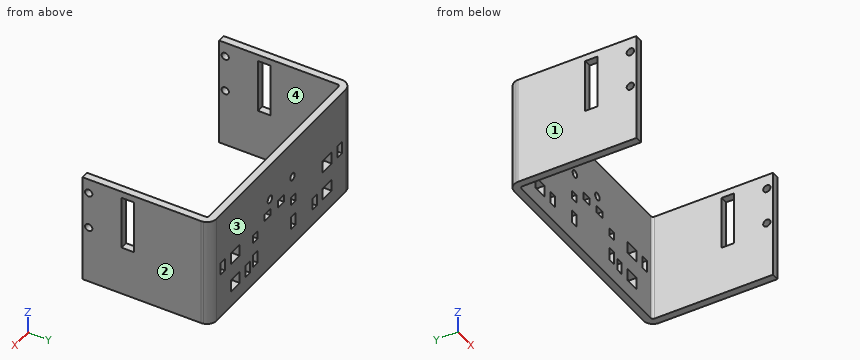
from build123d import *

# Parameters (mm, degrees)
SKETCH1_R                  = 1.5
SKETCH1_W                  = 2.9
SKETCH1_H                  = 5
SKETCH1_W_2                = 6
SKETCH1_W_3                = 5
SKETCH1_H_2                = 22
BASE_FLANGE1_DEPTH         = 3
SKETCH34_W                 = 3
SKETCH34_H                 = 5.190452684
SKETCH34_H_2               = 3.298760194
CUT_EXTRUDE2_DEPTH         = 10
SKETCH35_W                 = 4
SKETCH35_H                 = 3
CUT_EXTRUDE3_DEPTH         = 10
SKETCHED_START             = -31.946571622
SKETCHED_BEND1_DEPTH       = 45
SKETCHED_BEND1_2_OUTLINE_W = 3
SKETCHED_BEND1_2_OUTLINE_H = 16
SKETCHED_BEND1_2_DEPTH     = 45
SKETCHED_BEND1_3_OUTLINE_W = 3
SKETCHED_BEND1_3_OUTLINE_H = 5
SKETCHED_BEND1_3_DEPTH     = 20.3
SKETCHED_START_2           = 10.353428378
SKETCHED_BEND1_4_OUTLINE_W = 3
SKETCHED_BEND1_4_OUTLINE_H = 5
SKETCHED_BEND1_4_DEPTH     = 2.7
SKETCHED_START_3           = -48
SKETCHED_BEND1_5_OUTLINE_R = 1.5
SKETCHED_BEND1_5_DEPTH     = 96


with BuildPart() as part:
    # Base-Flange1: sheet metal written as solids
    # Sketch1 → Base-Flange1 (new body)
    with BuildSketch(Plane(origin=(0, 0, 0), x_dir=(1, 0, 0), z_dir=(0, 1, 0))):
        Polygon((-95, 31.946571622), (-95, -13.053428378), (95, -13.053428378), (95, 31.946571622), (45, 31.946571622), (-45, 31.946571622), align=None)
        with Locations(Location((92.5, -7.053428378, 0), (0, 0, 270))):
            Circle(SKETCH1_R, mode=Mode.SUBTRACT)
        with Locations(Location((92.5, 8.146571622, 0), (0, 0, 270))):
            Circle(SKETCH1_R, mode=Mode.SUBTRACT)
        with Locations(Location((-92.5, -7.053428378, 0), (0, 0, 90))):
            Circle(SKETCH1_R, mode=Mode.SUBTRACT)
        with Locations(Location((-92.5, 8.146571622, 0), (0, 0, 90))):
            Circle(SKETCH1_R, mode=Mode.SUBTRACT)
        with Locations(Location((7.6, 1.946571622, 0), (0, 0, 270))):
            Circle(SKETCH1_R, mode=Mode.SUBTRACT)
        with Locations(Location((-7.6, 1.946571622, 0), (0, 0, 270))):
            Circle(SKETCH1_R, mode=Mode.SUBTRACT)
        with Locations((-39.45, 10.905641405)):
            Rectangle(SKETCH1_W, SKETCH1_H, mode=Mode.SUBTRACT)
        with Locations((-22.55, 22.947848405)):
            Rectangle(SKETCH1_W, SKETCH1_H, mode=Mode.SUBTRACT)
        with Locations((-31, 22.946571622)):
            Rectangle(SKETCH1_W_2, SKETCH1_H, mode=Mode.SUBTRACT)
        with Locations((-31, 10.946571622)):
            Rectangle(SKETCH1_W_2, SKETCH1_H, mode=Mode.SUBTRACT)
        with Locations((31, 10.946571622)):
            Rectangle(SKETCH1_W_2, SKETCH1_H, mode=Mode.SUBTRACT)
        with Locations((31, 22.946571622)):
            Rectangle(SKETCH1_W_2, SKETCH1_H, mode=Mode.SUBTRACT)
        with Locations((22.55, 22.947848405)):
            Rectangle(SKETCH1_W, SKETCH1_H, mode=Mode.SUBTRACT)
        with Locations((39.45, 10.905641405)):
            Rectangle(SKETCH1_W, SKETCH1_H, mode=Mode.SUBTRACT)
        with Locations((76.5, 0.646571622)):
            Rectangle(SKETCH1_W_3, SKETCH1_H_2, mode=Mode.SUBTRACT)
        with Locations((-76.5, 0.646571622)):
            Rectangle(SKETCH1_W_3, SKETCH1_H_2, mode=Mode.SUBTRACT)
    extrude(amount=-BASE_FLANGE1_DEPTH)

    # Sketch34 → Cut-Extrude2 (cut)
    with BuildSketch(Plane.XZ.offset(3)):
        with Locations((17.4, -21.824895141)):
            Rectangle(SKETCH34_W, SKETCH34_H)
        with Locations((-8.1, -21.824895141)):
            Rectangle(SKETCH34_W, SKETCH34_H)
        with Locations((-8.1, -12.169238167)):
            Rectangle(SKETCH34_W, SKETCH34_H_2)
        with Locations((17.4, -12.169238167)):
            Rectangle(SKETCH34_W, SKETCH34_H_2)
    extrude(amount=-CUT_EXTRUDE2_DEPTH, mode=Mode.SUBTRACT)

    # Sketch35 → Cut-Extrude3 (cut)
    with BuildSketch(Plane(origin=(0, 0, 0), x_dir=(1, 0, 0), z_dir=(0, 1, 0))):
        with Locations((0.15, 7.74985807)):
            Rectangle(SKETCH35_W, SKETCH35_H)
        with Locations((9.15, 7.806187778)):
            Rectangle(SKETCH35_W, SKETCH35_H)
    extrude(amount=-CUT_EXTRUDE3_DEPTH, mode=Mode.SUBTRACT)

    # Sketched Bend1: read off the stored shape, not the designer's step
    # Sketched Bend1 outline → Sketched Bend1 (cut)
    with BuildSketch(Plane.XY.offset(SKETCHED_START)):
        with BuildLine():
            ThreePointArc((43.5, 0), (45.949489743, -0.83772234), (47.372983346, -3))
            Line((47.372983346, -3), (95, -3))
            Line((95, -3), (95, 0))
            Line((95, 0), (43.5, 0))
        make_face()
        with BuildLine():
            ThreePointArc((-47.372983346, -3), (-45.949489743, -0.83772234), (-43.5, 0))
            Line((-43.5, 0), (-95, 0))
            Line((-95, 0), (-95, -3))
            Line((-95, -3), (-47.372983346, -3))
        make_face()
    extrude(amount=SKETCHED_BEND1_DEPTH, mode=Mode.SUBTRACT)

    # Sketched Bend1 2 outline → Sketched Bend1 2 (add)
    with BuildSketch(Plane.XY.offset(SKETCHED_START)):
        with BuildLine():
            ThreePointArc((43.5, -3), (44.207106781, -3.292893219), (44.5, -4))
            Line((44.5, -4), (44.5, -31.5))
            Line((44.5, -31.5), (47.5, -31.5))
            Line((47.5, -31.5), (47.5, -4))
            ThreePointArc((47.5, -4), (47.468118785, -3.49598283), (47.372983346, -3))
            Line((47.372983346, -3), (43.5, -3))
        make_face()
        with BuildLine():
            ThreePointArc((-44.5, -4), (-44.207106781, -3.292893219), (-43.5, -3))
            Line((-43.5, -3), (-47.372983346, -3))
            ThreePointArc((-47.372983346, -3), (-47.468118785, -3.49598283), (-47.5, -4))
            Line((-47.5, -4), (-47.5, -31.5))
            Line((-47.5, -31.5), (-44.5, -31.5))
            Line((-44.5, -31.5), (-44.5, -4))
        make_face()
        with Locations((46, -44.5)):
            Rectangle(SKETCHED_BEND1_2_OUTLINE_W, SKETCHED_BEND1_2_OUTLINE_H)
        with Locations((-46, -44.5)):
            Rectangle(SKETCHED_BEND1_2_OUTLINE_W, SKETCHED_BEND1_2_OUTLINE_H)
    extrude(amount=SKETCHED_BEND1_2_DEPTH)

    # Sketched Bend1 3 outline → Sketched Bend1 3 (add)
    with BuildSketch(Plane.XY.offset(SKETCHED_START)):
        with Locations((46, -34)):
            Rectangle(SKETCHED_BEND1_3_OUTLINE_W, SKETCHED_BEND1_3_OUTLINE_H)
        with Locations((-46, -34)):
            Rectangle(SKETCHED_BEND1_3_OUTLINE_W, SKETCHED_BEND1_3_OUTLINE_H)
    extrude(amount=SKETCHED_BEND1_3_DEPTH)

    # Sketched Bend1 4 outline → Sketched Bend1 4 (add)
    with BuildSketch(Plane.XY.offset(SKETCHED_START_2)):
        with Locations((46, -34)):
            Rectangle(SKETCHED_BEND1_4_OUTLINE_W, SKETCHED_BEND1_4_OUTLINE_H)
        with Locations((-46, -34)):
            Rectangle(SKETCHED_BEND1_4_OUTLINE_W, SKETCHED_BEND1_4_OUTLINE_H)
    extrude(amount=SKETCHED_BEND1_4_DEPTH)

    # Sketched Bend1 5 outline → Sketched Bend1 5 (cut)
    with BuildSketch(Plane.YZ.offset(SKETCHED_START_3)):
        with Locations((-50, -8.146571622)):
            Circle(SKETCHED_BEND1_5_OUTLINE_R)
        with Locations((-50, 7.053428378)):
            Circle(SKETCHED_BEND1_5_OUTLINE_R)
    extrude(amount=SKETCHED_BEND1_5_DEPTH, mode=Mode.SUBTRACT)


solid = part.part
CAD build for the part. Positions are in the model's coordinates, mm. Face numbers are marked on the shaded views. Coordinates: 2 decimals unless noted, no trailing zeros. Loops run counter-clockwise (first coordinate to the right, second up) from the corner with the lowest first, then second, coordinate; pieces in that order, holes last. Notation, with made-up numbers: (-34.5, 84) -> (-19.5, 84) arc R14 cw to (-19.5, 107) -> close; hole circle Ø10 at (74.25, 89.5). An arc over 180 degrees is marked (long way). One line per item, written item: value.
1. Slice it at B-B on y = -50. Write the cut outline in (x, z), and give its area (3 significant figures).
Answers:
outline: (-47.5, -31.95) -> (-44.5, -31.95) -> (-44.5, -9.65) -> (-47.5, -9.65) -> close; (-47.5, -6.65) -> (-44.5, -6.65) -> (-44.5, 5.55) -> (-47.5, 5.55) -> close; (-47.5, 8.55) -> (-44.5, 8.55) -> (-44.5, 13.05) -> (-47.5, 13.05) -> close; (44.5, -31.95) -> (47.5, -31.95) -> (47.5, -9.65) -> (44.5, -9.65) -> close; (44.5, -6.65) -> (47.5, -6.65) -> (47.5, 5.55) -> (44.5, 5.55) -> close; (44.5, 8.55) -> (47.5, 8.55) -> (47.5, 13.05) -> (44.5, 13.05) -> close
area: 234 mm^2
2. Slice it at C-C on x = 0. Write the cut outline in (y, z), and give its area (3 significant figures).
Answers:
outline: (-3, -31.95) -> (0, -31.95) -> (0, -9.25) -> (-3, -9.25) -> close; (-3, -6.25) -> (0, -6.25) -> (0, 13.05) -> (-3, 13.05) -> close
area: 126 mm^2
3. Slice it at D-D on y = -24.5. Write the cut outline in (x, z).
Answers:
outline: (-47.5, -31.95) -> (-44.5, -31.95) -> (-44.5, 13.05) -> (-47.5, 13.05) -> close; (44.5, -31.95) -> (47.5, -31.95) -> (47.5, 13.05) -> (44.5, 13.05) -> close
4. Slice it at A-A on z = -4.5. Write the cut outline in (x, y), and give its area (3 significant figures).
Answers:
outline: (-47.5, -52.5) -> (-44.5, -52.5) -> (-44.5, -36.5) -> (-47.5, -36.5) -> close; (-47.5, -31.5) -> (-44.5, -31.5) -> (-44.5, -4) arc R1 cw to (-43.5, -3) -> (43.5, -3) arc R1 cw to (44.5, -4) -> (44.5, -31.5) -> (47.5, -31.5) -> (47.5, -4) arc R4 ccw to (43.5, 0) -> (-43.5, 0) arc R4 ccw to (-47.5, -4) -> close; (44.5, -52.5) -> (47.5, -52.5) -> (47.5, -36.5) -> (44.5, -36.5) -> close
area: 546 mm^2
5. Flat gauge pins, fed straight in: P1, Ø1, axis at x = -8.5, z = 4.5, coming from the -Y side; P2, Ø0.9, axis at x = -46.5, z = 3.5, coming from the +Y side; P3, Ø3.5, axis at y = -1.5, z = -22.5, coming from the -X side; P4, Ø12, axis at x = 3, y = -14.5, coming from the -Z side. Where does each tip first touch, or does it go through?
Answers:
P1: stops at y = -3
P2: stops at y = -0.92
P3: stops at x = -47.43
P4: passes through
6. Pull direction X, two halves, no side cores. Call the marked faces 1, 2, 3 and 4: pulls with the +X half, pulls with the -X half, needs draft (parallel to the pull), parting line crosses it, or undercut.
Answers:
face 1: pulls with the -X half
face 2: pulls with the +X half
face 3: needs draft
face 4: undercut
7. Drill centre lines: line 1 (Z direction, x = -46, y = -50); line 2 (X direction, y = -16, z = -27.5); line 3 (Y direction, x = 35.5, z = -28). Where is each one in solid material? Low to high. Write a range as [from, to].
Answers:
line 1: z = [-31.95, -9.65], [-6.65, 5.55], [8.55, 13.05]
line 2: x = [-47.5, -44.5], [44.5, 47.5]
line 3: y = [-3, 0]
